Geometry: final body of the model. Coordinates: model frame, mm. A direction names the side the tool comes from. Give positions to 0.01 mm unless a question says otherwise; leave off trailing zeros. Write each loop counter-clockwise with the first axis right and the second up, starting at its lowest first coordinate (ties: lowest second). Pieces come first, ordered by that corner, then holes.
Q1. Mould query, pull axis Z, two halves, no side actions, for faces 3 (the flat face through (-7, 0, 7)), 4 (the flat face through (-7, -10, 7)), 5 (the flat face through (-7, -153, -500)). Classes: +Z half, -Z half, draft (parallel to the pull), parting line (faces both ways), or undercut.
Q2. Section B-B (z = -116). Return the cut outline in (x, y).
Q3. Pin query (flat end, axial travel): pin 1 Ø8 at (x, z) = (-296.5, -187.5) entering from -Y. Return the tip coordinate at first contact, or that it passes through.
Q4. Section C-C (x = 418). Return the cut outline in (y, z), plus the area to 3 significant figures.
Q5. Reachability of faces 1 (the flat face through (-7, -158, 495)), 2 (the flat face through (500, -153, -7)) from +Z, -Z, +X, -X, +Y, -Y: full face, straight path, thin tool, end or side. Return the list, or none.
Q6. Line query: line 1 (X direction, y = -227.5, z = 166.5); line 2 (Y direction, x = -300.5, z = 201.5). Output: solid intervals per line, ascending.
Q7. Section A-A (y = -182). Return the cut outline in (x, z), plus the area to 3 significant figures.
from build123d import *

# Parameters (mm, degrees)
F0_W     = 1000
F0_H     = 1000
F1_DEPTH = 10
F2_W     = 990
F2_H     = 5
F3_DEPTH = 300


with BuildPart() as f1:
    # F0 (on Front) → F1 (new body)
    with BuildSketch(Plane.XZ):
        Rectangle(F0_W, F0_H)
    extrude(amount=F1_DEPTH)

    # F2 (on face) → F3 (join)
    with BuildSketch(Plane.XZ.offset(10)):
        Polygon((-495, 500), (-500, 500), (-500, -500), (-495, -500), (-495, -495), (-495, 495), align=None)
        Polygon((500, 500), (-495, 500), (-495, 495), (495, 495), (500, 495), align=None)
        with Locations((0, -497.5)):
            Rectangle(F2_W, F2_H)
        Polygon((500, 495), (495, 495), (495, -495), (495, -500), (500, -500), align=None)
    extrude(amount=F3_DEPTH)


solid = f1.part
Computed:
1. face 3: draft
1. face 4: undercut
1. face 5: -Z half
2. outline: (-500, -310) - (-495, -310) - (-495, -10) - (495, -10) - (495, -310) - (500, -310) - (500, 0) - (-500, 0) - close
3. pin 1: stops at y = -10
4. outline: (-310, -500) - (0, -500) - (0, 500) - (-310, 500) - (-310, 495) - (-10, 495) - (-10, -495) - (-310, -495) - close
4. area: 13,000 mm2
5. face 1: -Y
5. face 2: +Z, -Z, +X, +Y, -Y
6. line 1: x = -500 to -495, 495 to 500
6. line 2: y = -10 to 0
7. outline: (-500, -500) - (500, -500) - (500, 500) - (-500, 500) - close; hole (-495, -495) - (495, -495) - (495, 495) - (-495, 495) - close
7. area: 19,900 mm2
